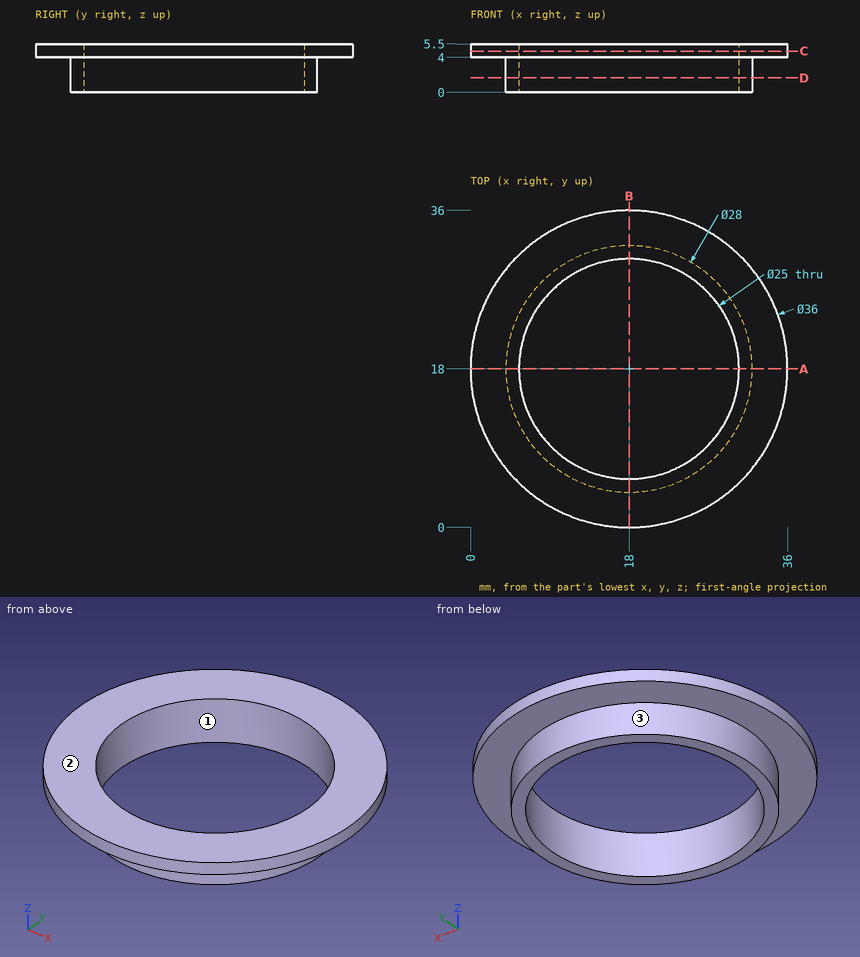
Could you check a few things on this drawing? It's one solid part, dimensions in mm from its lowest x, y, z. Coordinates: 2 decimals unless noted, no trailing zeros. Write each loop counter-clockwise with the first axis right and the second up, starting at its lowest first coordinate (ties: lowest second). Pieces come first, ordered by that corner, then holes.
Q1. Imagine slicing it at A-A, the plane y = 18. List the corners of the cut face in (x, z) for me, plus the area to 3 significant figures.
Results found:
outline: (0, 4) - (4, 4) - (4, 0) - (5.5, 0) - (5.5, 5.5) - (0, 5.5) - close; (30.5, 0) - (32, 0) - (32, 4) - (36, 4) - (36, 5.5) - (30.5, 5.5) - close
area: 28.5 mm2
Q2. Please list where these lines run through material, in increasing order: L1, parallel to Y at x = 18, z = 4.2; L2, parallel to Y at x = 18, z = 2.1; L3, parallel to X at y = 19, z = 4.3.
Results found:
L1: y = 0 to 5.5, 30.5 to 36
L2: y = 4 to 5.5, 30.5 to 32
L3: x = 0.03 to 5.54, 30.46 to 35.97
Q3. If we mould it in two halves opening along Y, with no side actions, what happens to the marked faces 1, 2 and 3? For each: +Y half, -Y half, draft (parallel to the pull), parting line (faces both ways), or undercut.
Results found:
face 1: undercut
face 2: draft
face 3: parting line
Q4. Imagine slicing it at D-D, the plane z = 1.65. List the corners of the cut face in (x, y) for me.
Results found:
outline: circle Ø28 at (18, 18); hole circle Ø25 at (18, 18)
Q5. Imagine slicing it at C-C, the plane z = 4.7. List the corners of the cut face in (x, y) for me, plus the area to 3 significant figures.
Results found:
outline: circle Ø36 at (18, 18); hole circle Ø25 at (18, 18)
area: 527 mm2
Q6. For P1, Ø2, axis at y = 8, z = 1, coming from the -X side; P2, Ø1, axis at y = 6.5, z = 5, coming from the -X side; P3, Ø3, axis at x = 19.5, z = 2, coming from the -Y side; P4, Ø11, axis at x = 21.5, y = 20.5, coming from the -Z side, each with a flat end and sliding along its axis, tell me the tip position at first contact or that it passes through.
Results found:
P1: stops at x = 7.28
P2: stops at x = 3.75
P3: stops at y = 4
P4: passes through
